from build123d import *

# Parameters (mm, degrees)
SKETCH2_W           = 101.6
SKETCH2_H           = 53.34
BOSS_EXTRUDE1_DEPTH = 1.14
SKETCH3_R           = 1.6
CUT_EXTRUDE1_DEPTH  = 115.756329673
SKETCH4_W           = 20.59
SKETCH4_H           = 3.2
SKETCH4_W_2         = 16.256
BOSS_EXTRUDE2_DEPTH = 9
CUT_EXTRUDE2_DEPTH  = 116.10306512
SKETCH6_R           = 1.6
CUT_EXTRUDE3_DEPTH  = 116.10306512
SKETCH7_W           = 3.245231175
SKETCH7_H           = 45.43323645
BOSS_EXTRUDE3_DEPTH = 9
SKETCH8_W           = 16.51
SKETCH8_H           = 10.150135712
SKETCH8_W_2         = 13.97
SKETCH8_H_2         = 8.650400862
BOSS_EXTRUDE4_DEPTH = 11.36
SKETCH9_R           = 3.217681585
SKETCH9_R_2         = 1.182707285
CUT_EXTRUDE4_DEPTH  = 11.36
SKETCH10_W          = 6.35
SKETCH10_H          = 5.56209116
SKETCH10_W_2        = 5.200759748
SKETCH10_H_2        = 1.452464435
CUT_EXTRUDE5_DEPTH  = 11.36
CHAMFER1_SIZE       = 1.524
SKETCH11_W          = 6.176206758
SKETCH11_H          = 7.62
BOSS_EXTRUDE5_DEPTH = 0.635
SKETCH12_W          = 8.456815018
SKETCH12_H          = 0.915706085
BOSS_EXTRUDE6_DEPTH = 0.254
FILLET1_R           = 0.508


with BuildPart() as part:
    # Sketch2 → Boss-Extrude1 (new body)
    with BuildSketch(Plane(origin=(0, 0, 0), x_dir=(1, 0, 0), z_dir=(0, 1, 0))):
        with Locations((50.8, 26.67)):
            Rectangle(SKETCH2_W, SKETCH2_H)
    extrude(amount=BOSS_EXTRUDE1_DEPTH)

    # Sketch3 → Cut-Extrude1 (cut, through all)
    with BuildSketch(Plane(origin=(0, 1.14, 0), x_dir=(1, 0, 0), z_dir=(0, 1, 0))):
        with Locations(Location((15.24, 50.8, 0), (0, 0, 270))):
            Circle(SKETCH3_R)
        with Locations(Location((15.24, 2.54, 0), (0, 0, 90))):
            Circle(SKETCH3_R)
    extrude(amount=-CUT_EXTRUDE1_DEPTH, mode=Mode.SUBTRACT)

    # Sketch4 → Boss-Extrude2 (add)
    with BuildSketch(Plane(origin=(0, 1.14, 0), x_dir=(1, 0, 0), z_dir=(0, 1, 0))):
        with Locations((56.015, 50.47)):
            Rectangle(SKETCH4_W, SKETCH4_H)
        with Locations((34.425, 50.47)):
            Rectangle(SKETCH4_W, SKETCH4_H)
        with Locations((78.875, 50.47)):
            Rectangle(SKETCH4_W, SKETCH4_H)
        with Locations((83.955, 2.87)):
            Rectangle(SKETCH4_W, SKETCH4_H)
        with Locations((61.095, 2.87)):
            Rectangle(SKETCH4_W, SKETCH4_H)
        with Locations((41.148, 2.87)):
            Rectangle(SKETCH4_W_2, SKETCH4_H)
    extrude(amount=BOSS_EXTRUDE2_DEPTH)

    # Sketch5 → Cut-Extrude2 (cut, through all)
    with BuildSketch(Plane(origin=(0, 1.14, 0), x_dir=(1, 0, 0), z_dir=(0, 1, 0))):
        Polygon((99.06, 0), (101.6, 0), (101.6, 2.54), align=None)
        Polygon((99.06, 41.584296227), (101.6, 39.37), (101.6, 53.321621524), (101.6, 53.34), (96.536046111, 53.34), (96.536046111, 53.321621524), (99.06, 51.121313818), align=None)
    extrude(amount=-CUT_EXTRUDE2_DEPTH, mode=Mode.SUBTRACT)

    # Sketch6 → Cut-Extrude3 (cut, through all)
    with BuildSketch(Plane(origin=(0, 1.14, 0), x_dir=(1, 0, 0), z_dir=(0, 1, 0))):
        with Locations(Location((96.52, 2.54, 0), (0, 0, 270))):
            Circle(SKETCH6_R)
        with Locations(Location((91.44, 50.8, 0), (0, 0, 270))):
            Circle(SKETCH6_R)
    extrude(amount=-CUT_EXTRUDE3_DEPTH, mode=Mode.SUBTRACT)

    # Sketch7 → Boss-Extrude3 (add)
    with BuildSketch(Plane(origin=(0, 1.14, 0), x_dir=(1, 0, 0), z_dir=(0, 1, 0))):
        with Locations((95.826679511, 29.119940639)):
            Rectangle(SKETCH7_W, SKETCH7_H)
    extrude(amount=BOSS_EXTRUDE3_DEPTH)

    # Sketch8 → Boss-Extrude4 (add)
    with BuildSketch(Plane(origin=(0, 1.14, 0), x_dir=(1, 0, 0), z_dir=(0, 1, 0))):
        with Locations((1.785, 37.873809091)):
            Rectangle(SKETCH8_W, SKETCH8_H)
        with Locations((4.885, 11.42677262)):
            Rectangle(SKETCH8_W_2, SKETCH8_H_2)
    extrude(amount=BOSS_EXTRUDE4_DEPTH)

    # Sketch9 → Cut-Extrude4 (cut)
    with BuildSketch(Plane.ZY.offset(2.1)):
        with Locations((-11.42677262, 7.870480003)):
            Circle(SKETCH9_R)
        with Locations((-11.42677262, 7.870480003)):
            Circle(SKETCH9_R_2, mode=Mode.SUBTRACT)
    extrude(amount=-CUT_EXTRUDE4_DEPTH, mode=Mode.SUBTRACT)

    # Sketch10 → Cut-Extrude5 (cut)
    with BuildSketch(Plane.ZY.offset(6.47)):
        with Locations((-37.873809091, 6.856773581)):
            Rectangle(SKETCH10_W, SKETCH10_H)
        with Locations((-37.84018947, 5.332133236)):
            Rectangle(SKETCH10_W_2, SKETCH10_H_2, mode=Mode.SUBTRACT)
    extrude(amount=-CUT_EXTRUDE5_DEPTH, mode=Mode.SUBTRACT)

    # Chamfer1
    chamfer1_edges = [part.edges().sort_by_distance(p)[0] for p in [
        (-0.79, 9.637819161, -41.048809091),
        (-0.79, 9.637819161, -34.698809091),
    ]]
    chamfer(chamfer1_edges, length=CHAMFER1_SIZE)

    # Sketch11 → Boss-Extrude5 (add)
    with BuildSketch(Plane(origin=(0, 1.14, 0), x_dir=(1, 0, 0), z_dir=(0, 1, 0))):
        with Locations((66.718103379, 28.71)):
            Rectangle(SKETCH11_W, SKETCH11_H)
    extrude(amount=BOSS_EXTRUDE5_DEPTH)

    # Sketch12 → Boss-Extrude6 (add)
    with BuildSketch(Plane(origin=(0, 1.14, 0), x_dir=(1, 0, 0), z_dir=(0, 1, 0))):
        with Locations((66.71021047, 28.609003409)):
            Rectangle(SKETCH12_W, SKETCH12_H)
        with Locations((66.71021047, 30.895003409)):
            Rectangle(SKETCH12_W, SKETCH12_H)
        with Locations((66.71021047, 26.323003408)):
            Rectangle(SKETCH12_W, SKETCH12_H)
    extrude(amount=BOSS_EXTRUDE6_DEPTH)

    # Fillet1
    # the kernel refuses this fillet: 0.508 mm, written as the material it takes off along each edge
    with BuildSketch(Plane(origin=(69.806206758, 1.775, -33.79), x_dir=(0, -1, 0), z_dir=(0, 0, 1))) as fillet1_piece_1_section:
        with BuildLine():
            CenterArc((FILLET1_R, -FILLET1_R), FILLET1_R, 90, 90)
            Line((0, -FILLET1_R), (0, 0))
            Line((0, 0), (FILLET1_R, 0))
        make_face()
    fillet1_piece_1 = extrude(amount=10.16, mode=Mode.PRIVATE)
    fillet1_piece_1 = split(fillet1_piece_1, bisect_by=Plane(origin=(69.801380886, 1.362351692, -31.352856451), z_dir=(0, 0, -1)), keep=Keep.TOP, mode=Mode.PRIVATE)
    add(fillet1_piece_1, mode=Mode.SUBTRACT)
    with BuildSketch(Plane(origin=(69.806206758, 1.775, -33.79), x_dir=(0, -1, 0), z_dir=(0, 0, 1))) as fillet1_piece_2_section:
        with BuildLine():
            CenterArc((FILLET1_R, -FILLET1_R), FILLET1_R, 90, 90)
            Line((0, -FILLET1_R), (0, 0))
            Line((0, 0), (FILLET1_R, 0))
        make_face()
    fillet1_piece_2 = extrude(amount=10.16, mode=Mode.PRIVATE)
    fillet1_piece_2 = split(fillet1_piece_2, bisect_by=Plane(origin=(69.691388297, 1.394, -30.895003408), z_dir=(0, 1, 0)), keep=Keep.TOP, mode=Mode.PRIVATE)
    add(fillet1_piece_2, mode=Mode.SUBTRACT)
    with BuildSketch(Plane(origin=(69.806206758, 1.775, -33.79), x_dir=(0, -1, 0), z_dir=(0, 0, 1))) as fillet1_piece_3_section:
        with BuildLine():
            CenterArc((FILLET1_R, -FILLET1_R), FILLET1_R, 90, 90)
            Line((0, -FILLET1_R), (0, 0))
            Line((0, 0), (FILLET1_R, 0))
        make_face()
    fillet1_piece_3 = extrude(amount=10.16, mode=Mode.PRIVATE)
    fillet1_piece_3 = split(fillet1_piece_3, bisect_by=Plane(origin=(69.801380886, 1.362351692, -29.066856451), z_dir=(0, 0, -1)), keep=Keep.TOP, mode=Mode.PRIVATE)
    fillet1_piece_3 = split(fillet1_piece_3, bisect_by=Plane(origin=(69.801380886, 1.362351692, -30.437150366), z_dir=(0, 0, 1)), keep=Keep.TOP, mode=Mode.PRIVATE)
    add(fillet1_piece_3, mode=Mode.SUBTRACT)
    with BuildSketch(Plane(origin=(69.806206758, 1.775, -33.79), x_dir=(0, -1, 0), z_dir=(0, 0, 1))) as fillet1_piece_4_section:
        with BuildLine():
            CenterArc((FILLET1_R, -FILLET1_R), FILLET1_R, 90, 90)
            Line((0, -FILLET1_R), (0, 0))
            Line((0, 0), (FILLET1_R, 0))
        make_face()
    fillet1_piece_4 = extrude(amount=10.16, mode=Mode.PRIVATE)
    fillet1_piece_4 = split(fillet1_piece_4, bisect_by=Plane(origin=(69.801380886, 1.362351692, -26.780856451), z_dir=(0, 0, -1)), keep=Keep.TOP, mode=Mode.PRIVATE)
    fillet1_piece_4 = split(fillet1_piece_4, bisect_by=Plane(origin=(69.801380886, 1.362351692, -28.151150366), z_dir=(0, 0, 1)), keep=Keep.TOP, mode=Mode.PRIVATE)
    add(fillet1_piece_4, mode=Mode.SUBTRACT)
    with BuildSketch(Plane(origin=(69.806206758, 1.775, -33.79), x_dir=(0, -1, 0), z_dir=(0, 0, 1))) as fillet1_piece_5_section:
        with BuildLine():
            CenterArc((FILLET1_R, -FILLET1_R), FILLET1_R, 90, 90)
            Line((0, -FILLET1_R), (0, 0))
            Line((0, 0), (FILLET1_R, 0))
        make_face()
    fillet1_piece_5 = extrude(amount=10.16, mode=Mode.PRIVATE)
    fillet1_piece_5 = split(fillet1_piece_5, bisect_by=Plane(origin=(69.801380886, 1.362351692, -25.865150366), z_dir=(0, 0, 1)), keep=Keep.TOP, mode=Mode.PRIVATE)
    add(fillet1_piece_5, mode=Mode.SUBTRACT)
    with BuildSketch(Plane(origin=(63.63, 1.775, -23.63), x_dir=(0, -1, 0), z_dir=(0, 0, -1))) as fillet1_piece_6_section:
        with BuildLine():
            CenterArc((FILLET1_R, -FILLET1_R), FILLET1_R, 90, 90)
            Line((0, -FILLET1_R), (0, 0))
            Line((0, 0), (FILLET1_R, 0))
        make_face()
    fillet1_piece_6 = extrude(amount=10.16, mode=Mode.PRIVATE)
    fillet1_piece_6 = split(fillet1_piece_6, bisect_by=Plane(origin=(63.634825872, 1.362351692, -25.865150366), z_dir=(0, 0, 1)), keep=Keep.TOP, mode=Mode.PRIVATE)
    add(fillet1_piece_6, mode=Mode.SUBTRACT)
    with BuildSketch(Plane(origin=(63.63, 1.775, -23.63), x_dir=(0, -1, 0), z_dir=(0, 0, -1))) as fillet1_piece_7_section:
        with BuildLine():
            CenterArc((FILLET1_R, -FILLET1_R), FILLET1_R, 90, 90)
            Line((0, -FILLET1_R), (0, 0))
            Line((0, 0), (FILLET1_R, 0))
        make_face()
    fillet1_piece_7 = extrude(amount=10.16, mode=Mode.PRIVATE)
    fillet1_piece_7 = split(fillet1_piece_7, bisect_by=Plane(origin=(63.744818461, 1.394, -26.323003408), z_dir=(0, 1, 0)), keep=Keep.TOP, mode=Mode.PRIVATE)
    add(fillet1_piece_7, mode=Mode.SUBTRACT)
    with BuildSketch(Plane(origin=(63.63, 1.775, -23.63), x_dir=(0, -1, 0), z_dir=(0, 0, -1))) as fillet1_piece_8_section:
        with BuildLine():
            CenterArc((FILLET1_R, -FILLET1_R), FILLET1_R, 90, 90)
            Line((0, -FILLET1_R), (0, 0))
            Line((0, 0), (FILLET1_R, 0))
        make_face()
    fillet1_piece_8 = extrude(amount=10.16, mode=Mode.PRIVATE)
    fillet1_piece_8 = split(fillet1_piece_8, bisect_by=Plane(origin=(63.634825872, 1.362351692, -28.151150366), z_dir=(0, 0, 1)), keep=Keep.TOP, mode=Mode.PRIVATE)
    fillet1_piece_8 = split(fillet1_piece_8, bisect_by=Plane(origin=(63.634825872, 1.362351692, -26.780856451), z_dir=(0, 0, -1)), keep=Keep.TOP, mode=Mode.PRIVATE)
    add(fillet1_piece_8, mode=Mode.SUBTRACT)
    with BuildSketch(Plane(origin=(63.63, 1.775, -23.63), x_dir=(0, -1, 0), z_dir=(0, 0, -1))) as fillet1_piece_9_section:
        with BuildLine():
            CenterArc((FILLET1_R, -FILLET1_R), FILLET1_R, 90, 90)
            Line((0, -FILLET1_R), (0, 0))
            Line((0, 0), (FILLET1_R, 0))
        make_face()
    fillet1_piece_9 = extrude(amount=10.16, mode=Mode.PRIVATE)
    fillet1_piece_9 = split(fillet1_piece_9, bisect_by=Plane(origin=(63.634825872, 1.362351692, -30.437150366), z_dir=(0, 0, 1)), keep=Keep.TOP, mode=Mode.PRIVATE)
    fillet1_piece_9 = split(fillet1_piece_9, bisect_by=Plane(origin=(63.634825872, 1.362351692, -29.066856451), z_dir=(0, 0, -1)), keep=Keep.TOP, mode=Mode.PRIVATE)
    add(fillet1_piece_9, mode=Mode.SUBTRACT)
    with BuildSketch(Plane(origin=(63.63, 1.775, -23.63), x_dir=(0, -1, 0), z_dir=(0, 0, -1))) as fillet1_piece_10_section:
        with BuildLine():
            CenterArc((FILLET1_R, -FILLET1_R), FILLET1_R, 90, 90)
            Line((0, -FILLET1_R), (0, 0))
            Line((0, 0), (FILLET1_R, 0))
        make_face()
    fillet1_piece_10 = extrude(amount=10.16, mode=Mode.PRIVATE)
    fillet1_piece_10 = split(fillet1_piece_10, bisect_by=Plane(origin=(63.634825872, 1.362351692, -31.352856451), z_dir=(0, 0, -1)), keep=Keep.TOP, mode=Mode.PRIVATE)
    add(fillet1_piece_10, mode=Mode.SUBTRACT)


solid = part.part
Work out the finished part from the listing and answer in its coordinate system (mm). A direction names the side the tool comes from. Give positions to 0.01 mm unless a question says otherwise; leave off trailing zeros. Write each loop counter-clockwise with the first axis right and the second up, starting at its lowest first coordinate (ties: lowest second). Pieces come first, ordered by that corner, then holes. Notation, with made-up numbers: (-10.75, 26) - (47.25, 26) arc R19 ccw to (47.25, 32) - close; hole circle Ø8 at (-21, 37). An arc over 180 degrees is marked (long way). One line per item, written item: value. Start each with the question number.
1. Find section C-C (z = -46). Write down the section's boundary in (x, y).
2. Consider probe 1 along X at (y, z) = (0.25, -2.54); probe 2 along X at (y, z) = (0.35, -50.8); probe 3 along Z at (x, y) = (77, 7.75). Determine where each line is inside the solid, lowest interval first.
3. For faces 4 (the flat face through (-1, 4.076, -38)), 5 (the flat face through (-3, 1.14, -38)), 6 (the flat face through (10.04, 7, -38)), 7 (the flat face through (5, 7, -7.102)), determine the directions among +Z, -Z, +X, -X, +Y, -Y from which every point of the face is accessible in a straight line to the end or side of a thin tool.
4. Find section A-A (x = 15.24). Write down the section's boundary in (y, z).
5. Given pin 1 (4 mm diameter, centred on x = 67.5, y = 9, fed in from +Z); pin 2 (1.6 mm diameter, centred on y = 6, z = -50, fed in from +X); pin 3 (4 mm diameter, centred on x = 30.5, y = 5.5, fed in from -Z), each flat-ended and moving along its own axis, determine where each tip first touches the part or whether it passes through.
6. Find section B-B (x = 91.44). Write down the section's boundary in (y, z).
7. Find section D-D (x = 38). Write down the section's boundary in (y, z).
8. For a pull along Z with two mould halves and no side action, classify faces 1 (the flat face through (84, 6, -4.47)), 2 (the flat face through (71.39, 6, -3)), 3 (the flat face through (97.78, 0.578, -52.237)) as +Z half, -Z half, draft (parallel to the pull), parting line (faces both ways), or undercut.
Geometry results:
1. outline: (0, 0) - (99.06, 0) - (99.06, 1.14) - (97.45, 1.14) - (97.45, 10.14) - (94.2, 10.14) - (94.2, 1.14) - (0, 1.14) - close
2. probe 1: 0 to 13.64, 16.84 to 94.92, 98.12 to 101.6
2. probe 2: 0 to 13.64, 16.84 to 89.84, 93.04 to 99.06
2. probe 3: -52.07 to -48.87, -4.47 to -1.27
3. face 4: -X
3. face 5: +Z, -Z, -X, -Y
3. face 6: -Z, +Y
3. face 7: +Z, -X, +Y
4. outline: (0, -53.34) - (1.14, -53.34) - (1.14, -52.4) - (0, -52.4) - close; (0, -49.2) - (1.14, -49.2) - (1.14, -4.14) - (0, -4.14) - close; (0, -0.94) - (1.14, -0.94) - (1.14, 0) - (0, 0) - close
5. pin 1: z = -1.27
5. pin 2: x = 97.45
5. pin 3: z = -52.07
6. outline: (0, -53.34) - (1.14, -53.34) - (1.14, -52.4) - (0, -52.4) - close; (0, -49.2) - (1.14, -49.2) - (1.14, -4.47) - (10.14, -4.47) - (10.14, -1.27) - (1.14, -1.27) - (1.14, 0) - (0, 0) - close
7. outline: (0, -53.34) - (1.14, -53.34) - (1.14, -52.07) - (10.14, -52.07) - (10.14, -48.87) - (1.14, -48.87) - (1.14, -4.47) - (10.14, -4.47) - (10.14, -1.27) - (1.14, -1.27) - (1.14, 0) - (0, 0) - close
8. face 1: undercut
8. face 2: draft
8. face 3: -Z half
